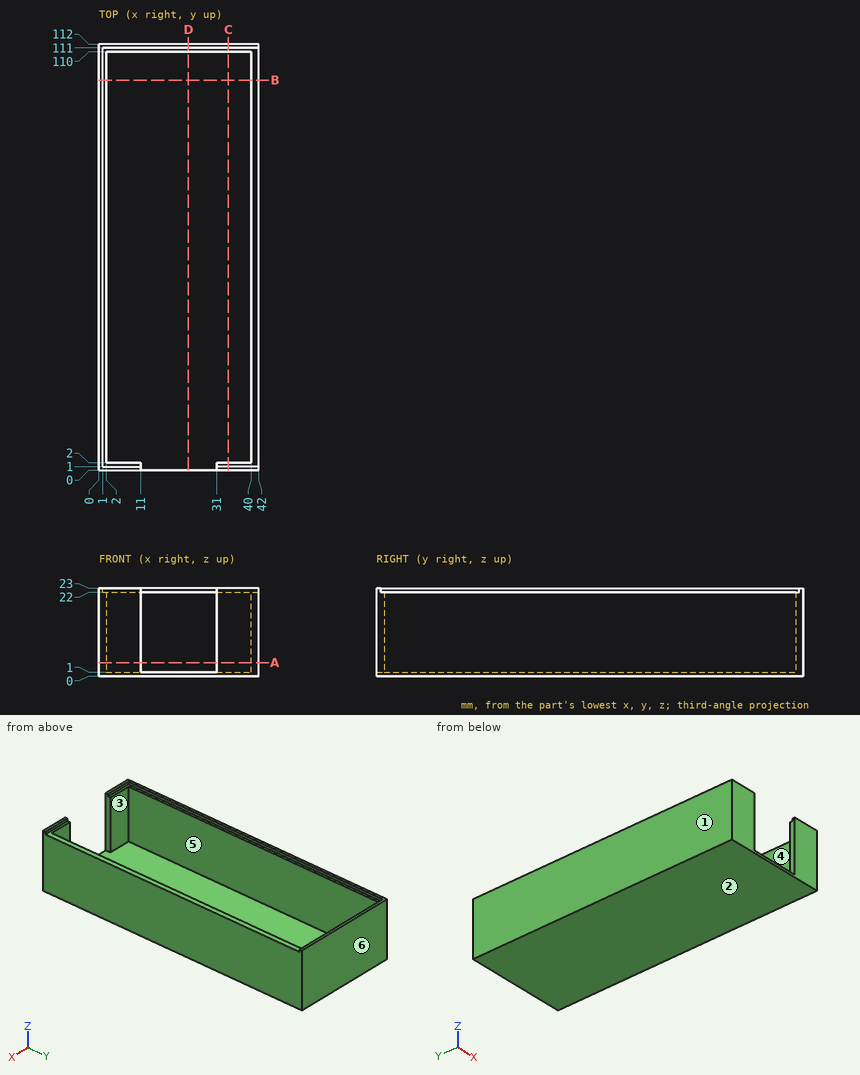
Job drawing, mm, ordinate dimensions from the low corner. One solid piece. A direction names the side the tool comes from. Round coordinates to 2 decimals unless told otherwise and drop trailing zeros. Loops run counter-clockwise (first coordinate to the right, second up) from the corner with the lowest first, then second, coordinate; pieces in that order, holes last. Notation, with made-up numbers: M -15.5,-6.75 L 42.5,-6.75 A16 cw 42.5,4.25 Z; hole C 57,-26 d8. An arc over 180 degrees is marked long. One line per question, with ' | ' between items. Start each with the question number.
Item 1: Cut at B-B, the plane y = 102.5. Write the cut outline in (x, z), plus the area to 3 significant figures.
Item 2: Cut at D-D, the plane x = 23.5. Write the cut outline in (y, z), plus the area to 3 significant figures.
Item 3: Wall check: line 1 (X direction, y = 50, z = 6); line 2 (Y direction, x = 33, z = 5.25); line 3 (Z direction, x = 30, y = 106). Give the ranges that are in metal, low to high.
Item 4: Which spindle directions (+Z, -Z, +X, -X, +Y, -Y) get a long thin tool onto all of the face, cutting with end or side? Do the marked faces 5 and 6. Say none if no direction does.
Item 5: Two-plate mould, pull along X, no slides. Class the marked faces 1, 2, 3 and 4: pulls with the +X half, pulls with the -X half, needs draft (parallel to the pull), parting line crosses it, or undercut.
Item 6: Cut at A-A, the plane z = 3.5. Write the cut outline in (x, y).
Item 7: Pin check, flat tips, straight feed: pin 1 Ø6.5 at (x, z) = (16.5, 14) entering from -Y; pin 2 Ø19 at (x, y) = (18, 28) entering from +Z; pin 3 Ø0.8 at (x, z) = (27.5, 22.5) entering from -Y. Stop position of each tip, or through.
Item 8: Cut at C-C, the plane x = 34. Write the cut outline in (y, z), plus the area to 3 significant figures.
Responses:
1) outline: M 0,0 L 42,0 L 42,22 L 40,22 L 40,1 L 2,1 L 2,22 L 1,22 L 1,23 L 0,23 Z | area: 127 mm²
2) outline: M 0,0 L 112,0 L 112,23 L 111,23 L 111,22 L 110,22 L 110,1 L 0,1 Z | area: 155 mm²
3) line 1: x = 0 to 2, 40 to 42 | line 2: y = 0 to 2, 110 to 112 | line 3: z = 0 to 1
4) face 5: +Z | face 6: +Z, -Z, +X, -X, +Y
5) face 1: pulls with the -X half | face 2: needs draft | face 3: undercut | face 4: undercut
6) outline: M 0,0 L 11,0 L 11,2 L 2,2 L 2,110 L 40,110 L 40,2 L 31,2 L 31,0 L 42,0 L 42,112 L 0,112 Z
7) pin 1: stops at y = 110 | pin 2: stops at z = 1 | pin 3: stops at y = 111
8) outline: M 0,0 L 112,0 L 112,23 L 111,23 L 111,22 L 110,22 L 110,1 L 2,1 L 2,22 L 1,22 L 1,23 L 0,23 Z | area: 198 mm²
